Work out the finished part from the listing and answer in its coordinate system (mm). Give positions to 0.01 mm unless a question says otherwise; leave off trailing zeros. Loops run counter-clockwise (first coordinate to the right, second up) from the corner with the lowest first, then second, coordinate; pieces in that order, holes last.
Autodesk Fusion 360 part; units mm, degrees
sketch "スケッチ1" plane through (0, 0, 0) normal (0, 0, 1) x (1, 0, 0)
  line L0 (10, -10) -> (-70, -10)
  line L1 (-70, -10) -> (-70, 0)
  line L2 (-70, 0) -> (10, 0)
  line L3 (10, 0) -> (10, -10)
extrude "押し出し1" add sketch "スケッチ1" along normal blind 20
sketch "スケッチ2" plane through (0, 0, 0) normal (0, 1, 0) x (-1, 0, 0)
  line L0 (-10, 0) -> (70, 0)
  line L1 (70, 0) -> (70, 20)
  line L2 (70, 20) -> (-10, 20)
  line L3 (-10, 20) -> (-10, 0)
  circle A0 centre (60, 10) radius 2.1
extrude "押し出し2" cut sketch "スケッチ2" against normal blind 10 contours A0
extrude "押し出し3" cut 1 faces at (-12.6333, -10, 10) along direction (0, 1, 0) blind 4
sketch "スケッチ3" plane through (0, 0, 0) normal (0, 1, 0) x (-1, 0, 0)
  circle A0 centre (60, 10) radius 2.1
  line L0 (-10, 0) -> (70, 0)
  line L1 (70, 0) -> (70, 20)
  line L2 (70, 20) -> (-10, 20)
  line L3 (-10, 20) -> (-10, 0)
  circle A1 centre (-5, 15) radius 1.5
  circle A2 centre (-5, 5) radius 1.5
extrude "押し出し4" cut sketch "スケッチ3" against normal blind 6 contours A1 | A2
Item 1: Find section D-D, the plane x = 5. Write down the section's boundary in (y, z), plus the area to 3 significant figures.
Item 2: Determine the mould class of faces 1 (the face through (6.2, -3, 4.1)), 2 (the face through (10, -3, 10)), 3 (the face through (-62.003, -2.958, 10.631)), 4 (the face through (-31, -3, 20)) for opening direction X: released by +X, released by -X, zero draft, split by the parting line, or undercut.
Item 3: A flat-ended cylindrical pin translates along its axis: pin 1 Ø2.5 at (x, z) = (5, 15) entering from +Y. Find the tip coordinate at first contact, or state that the pin passes through.
Item 4: Consider line 1 (Z direction, x = 5, y = -1.65); line 2 (Z direction, x = -60, y = -3); line 3 (Z direction, x = 6, y = -2.55). Determine where each line is inside the solid, lowest interval first.
Item 5: Find section C-C, the plane y = -4.4. Write down the section's boundary in (x, z), plus the area to 3 significant figures.
Item 6: Find section B-B, the plane x = -60. Write down the section's boundary in (y, z).
Item 7: Find section A-A, the plane z = 15. Write down the section's boundary in (x, y), plus the area to 3 significant figures.
Ans:
1. outline: (-6, 0) - (0, 0) - (0, 3.5) - (-6, 3.5) - close; (-6, 6.5) - (0, 6.5) - (0, 13.5) - (-6, 13.5) - close; (-6, 16.5) - (0, 16.5) - (0, 20) - (-6, 20) - close
1. area: 84.0 mm2
2. face 1: undercut
2. face 2: released by +X
2. face 3: undercut
2. face 4: zero draft
3. pin 1: passes through
4. line 1: z = 0 to 3.5, 6.5 to 13.5, 16.5 to 20
4. line 2: z = 0 to 7.9, 12.1 to 20
4. line 3: z = 0 to 3.88, 6.12 to 13.88, 16.12 to 20
5. outline: (-70, 0) - (10, 0) - (10, 20) - (-70, 20) - close; hole circle Ø4.2 at (-60, 10); hole circle Ø3 at (5, 5); hole circle Ø3 at (5, 15)
5. area: 1,570 mm2
6. outline: (-6, 0) - (0, 0) - (0, 7.9) - (-6, 7.9) - close; (-6, 12.1) - (0, 12.1) - (0, 20) - (-6, 20) - close
7. outline: (-70, -6) - (3.5, -6) - (3.5, 0) - (-70, 0) - close; (6.5, -6) - (10, -6) - (10, 0) - (6.5, 0) - close
7. area: 462 mm2
